Could you check a few things on this model? Use its own coordinates, in mm. Face numbers are marked on the shaded views. Give positions to 0.01 mm unless a question says otherwise; leave off trailing zeros. Write each loop counter-clockwise with the first axis right and the second up, starting at its lowest first coordinate (ties: lowest second). Pieces come first, ordered by that corner, then holes. Notation, with made-up numbers: (59, -27.5) - (68, -27.5) arc R7 ccw to (68, -21.5) - close; hole circle Ø4 at (25, -5.5). An arc over 180 degrees is marked (long way). Answer as CSV lines item,"result". Start each with the question number.
Q1. Will these pins go through, and if not, where does the flat tip stop? pin 1 Ø1 at (x, y) = (-3.5, 46) entering from +Z; pin 2 Ø12.5 at (x, z) = (0, 34.925) entering from +Y; pin 3 Ø5 at (x, y) = (17.5, 55) entering from +Z.
Q2. Imagine slicing it at D-D on y = 50. List the corners of the cut face in (x, z) for me.
Q3. We'd pull the mould along Y, two halves only. Please class the marked faces 1, 2 and 3: pulls with the +Y half, pulls with the -Y half, needs draft (parallel to the pull), parting line crosses it, or undercut.
Q4. Imagine slicing it at A-A on x = 0. State how many separate pieces and enclosed holes the cut face has, and give its area (3 significant figures).
Q5. Imagine slicing it at B-B on z = 0. List the corners of the cut face in (x, y) for me (3 decimals).
Q6. If I drill on line 1 along X through (y, z) = (52, 0.5); line 2 along Y through (x, z) = (-23.5, 21.5); line 3 along X through (y, z) = (48, -2.5), over which ranges is the centre line in solid material (lowest first)?
Q7. Imagine slicing it at C-C on y = 68.5. List the corners of the cut face in (x, z) for me, and give its area (3 significant figures).
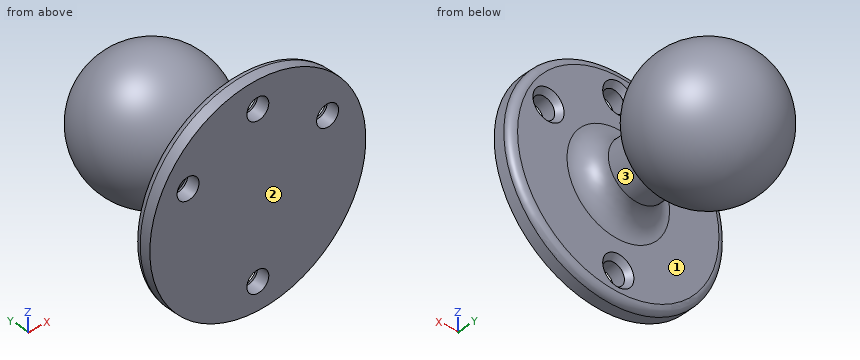
```python
from build123d import *

# Parameters (mm, degrees)
SKETCH3_R          = 4.7625
CUT_EXTRUDE1_DEPTH = 10
CHAMFER1_SIZE      = 2
CHAMFER1_SIZE2     = 2.383507185


with BuildPart() as part:
    # Sketch1 → Revolve1 (revolve)
    with BuildSketch(Plane(origin=(0, 0, 0), x_dir=(0, 0, -1), z_dir=(1, 0, 0))):
        with BuildLine():
            Line((0, 0), (46.8249, 0))
            Line((46.8249, 0), (46.8249, 4.7498))
            ThreePointArc((46.8249, 4.7498), (45.89496403, 6.99486403), (43.6499, 7.9248))
            Line((43.6499, 7.9248), (22.225, 7.9248))
            ThreePointArc((22.225, 7.9248), (15.489807909, 10.714607909), (12.7, 17.4498))
            Line((12.7, 17.4498), (12.7, 26.472331649))
            ThreePointArc((12.7, 26.472331649), (27.820711692, 58.592164207), (0, 80.645))
            Line((0, 80.645), (0, 0))
        make_face()
    revolve(axis=Axis((0, 0, 0), (0, 1, 0)))

    # Sketch3 → Cut-Extrude1 (cut)
    with BuildSketch(Plane.XZ):
        with Locations(Location((-30.2514, 17.4498, 0), (0, 0, 270))):
            Circle(SKETCH3_R)
        with Locations(Location((30.2514, 17.4498, 0), (0, 0, 270))):
            Circle(SKETCH3_R)
        with Locations(Location((0, -34.925, 0), (0, 0, 270))):
            Circle(SKETCH3_R)
        with Locations(Location((0, 34.925, 0), (0, 0, 270))):
            Circle(SKETCH3_R)
    extrude(amount=-CUT_EXTRUDE1_DEPTH, mode=Mode.SUBTRACT)

    # Chamfer1
    chamfer1_edges = [part.edges().sort_by_distance(p)[0] for p in [
        (-30.2514, 7.9248, 22.2123),
        (30.2514, 7.9248, 22.2123),
        (0, 7.9248, -30.1625),
        (0, 7.9248, 39.6875),
    ]]
    chamfer1_side = [part.faces().sort_by_distance(p)[0] for p in [
        (0, 7.9248, 42.415294388),
    ]]
    chamfer(chamfer1_edges, length=CHAMFER1_SIZE, length2=CHAMFER1_SIZE2, reference=chamfer1_side[0])


solid = part.part
```
Conclusion:
1,pin 1,"z = 27.82"
1,pin 2,"y = 7.31"
1,pin 3,"z = 24.17"
2,outline,"circle Ø57 at (0, 0)"
3,face 1,"undercut"
3,face 2,"pulls with the -Y half"
3,face 3,"undercut"
4,separate pieces,"3"
4,enclosed holes,"0"
4,area,"3,600 mm^2"
5,outline,"(-46.825, 0) - (46.825, 0) - (46.825, 4.75) arc R3.175 ccw to (43.65, 7.925) - (22.225, 7.925) arc R9.525 cw to (12.7, 17.45) - (12.7, 26.472) arc R28.575 ccw (long way) to (-12.7, 26.472) - (-12.7, 17.45) arc R9.525 cw to (-22.225, 7.925) - (-43.65, 7.925) arc R3.175 ccw to (-46.825, 4.75) - close"
6,line 1,"-28.57 to 28.57"
6,line 2,"0 to 7.92"
6,line 3,"-28.17 to 28.17"
7,outline,"circle Ø46.76 at (0, 0)"
7,area,"1,720 mm^2"
